```python
from build123d import *

# Parameters (mm, degrees)
SKETCH3_W          = 12.5
SKETCH3_H          = 12.6
CUT_EXTRUDE1_DEPTH = 10
CIRPATTERN1_COUNT  = 16
CUT_SWEEP3_ANGLE   = 46.890766
SKETCH8_R          = 27
SKETCH8_R_2        = 19.043703719
CUT_EXTRUDE2_DEPTH = 1.85


# Read off the part's stored shape, not the designer's step: Cut-Sweep3
with BuildPart() as part:
    # Sketch1 → Revolve1 (revolve)
    with BuildSketch(Plane(origin=(0, 0, 0), x_dir=(0, 0, -1), z_dir=(1, 0, 0))):
        Polygon((9.525, 0), (63.5, 0), (63.5, -15), (19.047086271, -15), (19.047086271, -34.735580232), (16.547086271, -34.735580232), (16.547086271, -37.235580232), (19.047086271, -37.235580232), (19.047086271, -40.235580232), (4.528779807, -52.235580232), (3.1, -52.235580232), (9.525, -40), align=None)
    revolve(axis=Axis((0, 0, 0), (0, 1, 0)))

    # Sketch3 → Cut-Extrude1 (cut)
    with BuildSketch(Plane(origin=(0, 0, 0), x_dir=(1, 0, 0), z_dir=(0, 1, 0))):
        with Locations((0, 50)):
            Rectangle(SKETCH3_W, SKETCH3_H)
    cut_extrude1 = extrude(amount=-CUT_EXTRUDE1_DEPTH, mode=Mode.SUBTRACT)

    # CirPattern1: Cut-Extrude1 ×16 about axis, 2 skipped
    cirpattern1_axis = Axis((0, 0, 0), (0, -1, 0))
    add([cut_extrude1.rotate(cirpattern1_axis, i * 360 / CIRPATTERN1_COUNT) for i in range(1, CIRPATTERN1_COUNT) if i not in (8, 9)], mode=Mode.SUBTRACT)

    # Cut-Sweep3 outline → Cut-Sweep3 (revolve, cut)
    with BuildSketch(Plane(origin=(0, 0, 0), x_dir=(-0.5705578043075098, 0, 0.8212574455941287), z_dir=(-0.8212574455941287, 0, -0.5705578043075098))):
        Polygon((54.406189133, -5), (54.406189133, 0), (9.525, 0), (9.525, -14.035371812), align=None)
    revolve(axis=Axis((0, 0, 0), (0, 1, 0)), revolution_arc=CUT_SWEEP3_ANGLE, mode=Mode.SUBTRACT)

    # Sketch8 → Cut-Extrude2 (cut)
    with BuildSketch(Plane.XZ.offset(15)):
        with Locations(Location((0, 0, 0), (0, 0, 270))):
            Circle(SKETCH8_R)
        with Locations(Location((0, 0, 0), (0, 0, 270))):
            Circle(SKETCH8_R_2, mode=Mode.SUBTRACT)
    extrude(amount=-CUT_EXTRUDE2_DEPTH, mode=Mode.SUBTRACT)


solid = part.part
```
Can you work these out from the model? Positions are in its coordinate system, mm. A direction names the side the tool comes from. Coordinates: 2 decimals unless noted, no trailing zeros. Write each loop counter-clockwise with the first axis right and the second up, starting at its lowest first coordinate (ties: lowest second). Pieces come first, ordered by that corner, then holes. Notation, with made-up numbers: M -30,0.5 L -1,0.5 A30 cw -1,37.5 Z; hole C -7,50.5 d4. An arc over 180 degrees is marked long. Answer as CSV lines item,"result".
Item 1: On a 3-axis mill with a long thin cutter (end or side, diameter ignored), from which of +Z, -Z, +X, -X, +Y, -Y can I reach the whole of each face in a straight line? I mean faces 4 (the flat face through (-52.05, -4.93, -21.46)), 5 (the cylindrical face through (18.6, -38.8, 4.1)), 6 (the cylindrical face through (61.99, -7.6, 13.77)). Say none if no direction works.
Geometry results:
face 4,"+Y"
face 5,"-Y"
face 6,"+Y, -Y"
Item 2: We'd pull the mould along Z, two halves only. Please class faces 1 (the flat face through (13, 0, -1)), 2 (the conical face through (5.109, -51.653, 1.135)), 3 (the cylindrical face through (-2.861, -19.72, -9.085)): +Z half, -Z half, draft (parallel to the pull), parting line (faces both ways), or undercut.
Geometry results:
face 1,"draft"
face 2,"parting line"
face 3,"undercut"
Item 3: Imagine slicing it at A-A on y = -47.5. List the corners of the cut face in (x, z) for me.
Geometry results:
outline,"C 0,0 d20.52; hole C 0,0 d11.17"
Item 4: I'm going to push flat-ended pins straight in: P1, Ø10, axis at y = -36.5, z = 8.5, coming from the -X side; P2, Ø5, axis at x = 10, z = -42.5, coming from the -Y side; P3, Ø1, axis at x = -2.5, z = -20.5, coming from the -Y side. Where does each tip first touch, or does it pass through?
Geometry results:
P1,"stops at x = -18.71"
P2,"stops at y = -15"
P3,"stops at y = -13.15"
Item 5: Please list where these lines run through material, in increasing order: line 1 along X through (y, z) = (-14.4, 0) (3 decimals); line 2 along Z through (x, y) = (0, -31) (3 decimals); line 3 along Z through (x, y) = (46, -1.5) (3 decimals).
Geometry results:
line 1,"x = -63.5 to -27, -19.044 to -9.525, 9.525 to 19.044, 27 to 63.5"
line 2,"z = -19.047 to -9.525, 9.525 to 19.047"
line 3,"z = -43.775 to -25.819, -12.289 to -6.25, 6.25 to 12.289, 25.819 to 43.775"
